Can you work these out from the model? Positions are in its coordinate system, mm. A direction names the side the tool comes from. Coordinates: 2 decimals unless noted, no trailing zeros. Order: outer loops, then holes, each group sorted by start corner. A loop starts at its lowest first (then second) coordinate and runs counter-clockwise, first axis right, second up. Notation, with made-up numbers: (35.5, 21.5) - (56.5, 21.5) arc R15 ccw to (56.5, 37.5) - close; hole circle Ø9 at (-27, 84). An arc over 180 degrees is marked (long way). Use a Markdown table: item, result. Add a question column.
(1) On a 3-axis mill with a long thin cutter (end or side, diameter ignored), from which of +Z, -Z, +X, -X, +Y, -Y can I reach the whole of each face in a straight line? I mean faces 1 (the flat face through (22.45, -5, 1)), 2 (the flat face through (12, 7, 3)), 3 (the flat face through (2.55, -5, 1)). Say none if no direction works.
(2) If I drill on L1, parallel to Y at x = 23, z = 1; L2, parallel to X at y = -6, z = 0.45, over which ranges is the centre line in solid material (lowest first)? Write a range as [from, to].
(3) For pin 1 Ø5 at (x, y) = (2, 22) entering from -Z; pin 2 Ø0.8 at (x, z) = (0.5, 1) entering from -Y; pin 3 Ø1.5 at (y, z) = (-3.5, 1) entering from +X, each with a flat end and sliding along its axis, tell me the tip position at first contact or that it passes through.
(4) I want a section at B-B (x = 2). List the corners of the cut face in (y, z) for me, and give its area (3 significant figures).
(5) I want a section at C-C (y = 22). List the corners of the cut face in (x, z) for me.
(6) We'd pull the mould along Y, two halves only. Please class faces 4 (the flat face through (12, 7, 0)), 5 (the cylindrical face through (2, 8, 1)), 6 (the flat face through (1, 0, 1)), 7 (the cylindrical face through (21.89, 23.01, 1.48)): pulls with the +Y half, pulls with the -Y half, needs draft (parallel to the pull), parting line crosses it, or undercut.
(7) I want a section at A-A (z = 2.05). List the corners of the cut face in (x, y) for me, and give its area (3 significant figures).
```python
from build123d import *

# Parameters (mm, degrees)
SKETCH1_W           = 25
SKETCH1_H           = 24
SKETCH1_R           = 1.5
SKETCH1_W_2         = 19.9
SKETCH1_H_2         = 10
BOSS_EXTRUDE1_DEPTH = 3


with BuildPart() as part:
    # Sketch1 → Boss-Extrude1 (new body)
    # profile 1 of 2: a face of its own
    with BuildSketch(Plane.XY):
        with Locations((12.5, 12)):
            Rectangle(SKETCH1_W, SKETCH1_H)
        with Locations((23, 22)):
            Circle(SKETCH1_R, mode=Mode.SUBTRACT)
        with Locations((2, 22)):
            Circle(SKETCH1_R, mode=Mode.SUBTRACT)
        with Locations((23, 9.5)):
            Circle(SKETCH1_R, mode=Mode.SUBTRACT)
        with Locations((2, 9.5)):
            Circle(SKETCH1_R, mode=Mode.SUBTRACT)
    # profile 2 of 2: a face of its own
    with BuildSketch(Plane.XY):
        with Locations((12.5, -5)):
            Rectangle(SKETCH1_W_2, SKETCH1_H_2)
    extrude(amount=BOSS_EXTRUDE1_DEPTH)


solid = part.part
```
Answers follow:
| question | item | result |
|---|---|---|
| 1 | face 1 | +Z, -Z, +X, -Y |
| 1 | face 2 | +Z, +X, -X, +Y, -Y |
| 1 | face 3 | +Z, -Z, -X, -Y |
| 2 | L1 | y = [0, 8], [11, 20.5], [23.5, 24] |
| 2 | L2 | x = [2.55, 22.45] |
| 3 | pin 1 | stops at z = 0 |
| 3 | pin 2 | stops at y = 0 |
| 3 | pin 3 | stops at x = 22.45 |
| 4 | outline | (0, 0) - (8, 0) - (8, 3) - (0, 3) - close; (11, 0) - (20.5, 0) - (20.5, 3) - (11, 3) - close; (23.5, 0) - (24, 0) - (24, 3) - (23.5, 3) - close |
| 4 | area | 54.0 mm² |
| 5 | outline | (0, 0) - (0.5, 0) - (0.5, 3) - (0, 3) - close; (3.5, 0) - (21.5, 0) - (21.5, 3) - (3.5, 3) - close; (24.5, 0) - (25, 0) - (25, 3) - (24.5, 3) - close |
| 6 | face 4 | needs draft |
| 6 | face 5 | undercut |
| 6 | face 6 | pulls with the -Y half |
| 6 | face 7 | undercut |
| 7 | outline | (0, 0) - (2.55, 0) - (2.55, -10) - (22.45, -10) - (22.45, 0) - (25, 0) - (25, 24) - (0, 24) - close; hole circle Ø3 at (2, 9.5); hole circle Ø3 at (2, 22); hole circle Ø3 at (23, 9.5); hole circle Ø3 at (23, 22) |
| 7 | area | 771 mm² |
